Design review of the part built by this model. Coordinates are the model's own, in mm. A direction names the side the tool comes from. Coordinates: 2 decimals unless noted, no trailing zeros. Order: outer loops, then holes, each group sorted by start corner. A loop starts at its lowest first (then second) coordinate and runs counter-clockwise, first axis right, second up. Notation, with made-up numbers: M 85.25,24 L 135.25,24 A6 ccw 135.25,33 Z; hole C 84,9.5 d3. An arc over 180 degrees is marked long. Answer in a Markdown table with one row per item.
from build123d import *

# Parameters (mm, degrees)
F0_W      = 30
F0_H      = 45
F1_DEPTH  = 20
F2_W      = 6
F2_H      = 6
F3_DEPTH  = 1
F5_DEPTH  = 1
F6_W      = 1
F6_H      = 30
F7_DEPTH  = 30
F8_W      = 23
F8_H      = 23
F9_DEPTH  = 3
F10_W     = 23
F10_H     = 23
F11_DEPTH = 3
F12_W     = 42
F12_H     = 30
F13_DEPTH = 2
F14_R     = 8
F15_DEPTH = 8
F17_DEPTH = 15
F18_W     = 42
F18_H     = 22.5
F19_DEPTH = 14
F21_R     = 8
F22_DEPTH = 8
F23_DEPTH = 42
F24_DEPTH = 1
F25_R     = 8
F26_DEPTH = 8
F27_R     = 8
F28_DEPTH = 8
F29_W     = 6
F29_H     = 6
F30_DEPTH = 1
F31_W     = 42
F31_H     = 5
F32_DEPTH = 3


with BuildPart() as f1:
    # F0 (on Right) → F1 (new body, symmetric)
    with BuildSketch(Plane.YZ):
        Rectangle(F0_W, F0_H)
    extrude(amount=F1_DEPTH, both=True)

    # F2 (on face) → F3 (join, symmetric)
    with BuildSketch(Plane(origin=(-20, 0, 0), x_dir=(0, -1, 0), z_dir=(-1, 0, 0))):
        Polygon((-15, -7.5), (-15, -22.5), (15, -22.5), (15, -7.5), (4.0889219381, -7.5), (4.0889219381, 2.5), (-4.0889219381, 2.5), (-4.0889219381, -7.5), align=None)
        with Locations((-7.5, 10.5)):
            Rectangle(F2_W, F2_H)
        with Locations((7.5, 10.5)):
            Rectangle(F2_W, F2_H)
    extrude(amount=F3_DEPTH, both=True)

    # F4 (on face) → F5 (join, symmetric)
    with BuildSketch(Plane.YZ.offset(20)):
        Polygon((-4.0889219381, -7.5), (-15, -7.5), (-15, -22.5), (15, -22.5), (15, -7.5), (4.0889219381, -7.5), (4.0889219381, 2.5), (-4.0889219381, 2.5), align=None)
    extrude(amount=F5_DEPTH, both=True)

    # F6 (on face) → F7 (join)
    with BuildSketch(Plane(origin=(0, 15, 0), x_dir=(-1, 0, 0), z_dir=(0, 1, 0))):
        with Locations((20.5, 7.5)):
            Rectangle(F6_W, F6_H)
        Polygon((-21, -22.5), (21, -22.5), (21, -7.5), (20, -7.5), (20, 22.5), (-20, 22.5), (-20, -7.5), (-21, -7.5), align=None)
        with Locations((-20.5, 7.5)):
            Rectangle(F6_W, F6_H)
    extrude(amount=F7_DEPTH)

    # F8 (on face) → F9 (cut)
    with BuildSketch(Plane(origin=(-21, 0, 0), x_dir=(0, -1, 0), z_dir=(-1, 0, 0))):
        with Locations((-30, 7.5)):
            Rectangle(F8_W, F8_H)
    extrude(amount=-F9_DEPTH, mode=Mode.SUBTRACT)

    # F10 (on face) → F11 (cut)
    with BuildSketch(Plane.YZ.offset(21)):
        with Locations((30, 7.5)):
            Rectangle(F10_W, F10_H)
    extrude(amount=-F11_DEPTH, mode=Mode.SUBTRACT)

    # F12 (on face) → F13 (join)
    with BuildSketch(Plane.XY.offset(22.5)):
        with Locations((0, 30)):
            Rectangle(F12_W, F12_H)
    extrude(amount=F13_DEPTH)

    # F14 (on face) → F15 (cut)
    with BuildSketch(Plane(origin=(-21, 0, 0), x_dir=(0, -1, 0), z_dir=(-1, 0, 0))):
        with Locations((-27, -22.5)):
            Circle(F14_R)
    extrude(amount=-F15_DEPTH, mode=Mode.SUBTRACT)

    # F16 (on face) → F17 (join)
    with BuildSketch(Plane.XZ.offset(15)):
        Polygon((-21, 24.5194389681), (-21, -22.5), (21, -22.5), (21, 24.5022866875), align=None)
    extrude(amount=F17_DEPTH)

    # F18 (on face) → F19 (join)
    with BuildSketch(Plane.XZ.offset(30)):
        with Locations((0, -11.25)):
            Rectangle(F18_W, F18_H)
    extrude(amount=F19_DEPTH)

    # F21 (on face) → F22 (cut)
    with BuildSketch(Plane.YZ.offset(21)):
        with Locations((27, -22.5)):
            Circle(F21_R)
    extrude(amount=-F22_DEPTH, mode=Mode.SUBTRACT)

    # F20 (on face) → F23 (join)
    with BuildSketch(Plane(origin=(-21, 0, 0), x_dir=(0, -1, 0), z_dir=(-1, 0, 0))):
        Polygon((44, 0), (30, 24.5194389681), (30, 0), align=None)
    extrude(amount=-F23_DEPTH)

    # F2 (on face) → F24 (join)
    with BuildSketch(Plane(origin=(-20, 0, 0), x_dir=(0, -1, 0), z_dir=(-1, 0, 0))):
        Polygon((-15, -7.5), (-15, -22.5), (15, -22.5), (15, -7.5), (4.0889219381, -7.5), (4.0889219381, 2.5), (-4.0889219381, 2.5), (-4.0889219381, -7.5), align=None)
        with Locations((-7.5, 10.5)):
            Rectangle(F2_W, F2_H)
        with Locations((7.5, 10.5)):
            Rectangle(F2_W, F2_H)
    extrude(amount=F24_DEPTH)

    # F25 (on face) → F26 (cut)
    with BuildSketch(Plane(origin=(-21, 0, 0), x_dir=(0, -1, 0), z_dir=(-1, 0, 0))):
        with Locations((26, -22.5)):
            Circle(F25_R)
    extrude(amount=-F26_DEPTH, mode=Mode.SUBTRACT)

    # F27 (on face) → F28 (cut)
    with BuildSketch(Plane.YZ.offset(21)):
        with Locations((-28, -22.5)):
            Circle(F27_R)
    extrude(amount=-F28_DEPTH, mode=Mode.SUBTRACT)

    # F29 (on face) → F30 (join, symmetric)
    with BuildSketch(Plane.YZ.offset(20)):
        with Locations((-7.5, 10.5)):
            Rectangle(F29_W, F29_H)
        with Locations((7.5, 10.5)):
            Rectangle(F29_W, F29_H)
    extrude(amount=F30_DEPTH, both=True)

    # F31 (on face) → F32 (join)
    with BuildSketch(Plane.XZ.offset(44)):
        with Locations((0, -20)):
            Rectangle(F31_W, F31_H)
    extrude(amount=F32_DEPTH)


solid = f1.part
(1) Add section B-B, the plane z = -2.5. Give the boundary of the cut face in (x, y), and give its area (3 significant figures).
Return value:
| item | result |
|---|---|
| outline | M -21,-44 L 21,-44 L 21,-15 L 20,-15 L 20,-4.09 L 21,-4.09 L 21,4.09 L 20,4.09 L 20,15 L 21,15 L 21,18.5 L 18,18.5 L 18,41.5 L 21,41.5 L 21,45 L -21,45 L -21,41.5 L -18,41.5 L -18,18.5 L -21,18.5 L -21,15 L -20,15 L -20,4.09 L -21,4.09 L -21,-4.09 L -20,-4.09 L -20,-15 L -21,-15 Z |
| area | 3,560 mm2 |
(2) For line 1 along X through (y, z) = (35, 9); line 2 along Z through (x, y) = (-4, 41); line 3 along X through (y, z) = (-13.5, -6), list the stretches that pass through material, from the lowest coordinate up. Write a range as from..to.
Return value:
| item | result |
|---|---|
| line 1 | x = -18..18 |
| line 2 | z = -22.5..24.5 |
| line 3 | x = -20..20 |
(3) For faces 4 (the flat face through (20, 41.5, 7)), 5 (the flat face through (-20, 18.5, 7)), 6 (the flat face through (-13, -26, -19)), 7 (the flat face through (0, 15, 23)), 8 (the flat face through (13, -28, -19)), list the 3-axis set-ups (+Z, -Z, +X, -X, +Y, -Y) from which the entire face can be reached by the end or side of a thin tool; tool diameter is ignored.
Return value:
| item | result |
|---|---|
| face 4 | +X |
| face 5 | -X |
| face 6 | -Z, -X |
| face 7 | +Z |
| face 8 | -Z, +X |
(4) Add section D-D, the plane y = -1. Give the boundary of the cut face in (x, z), and give its area (3 significant figures).
Return value:
| item | result |
|---|---|
| outline | M -21,-22.5 L 21,-22.5 L 21,2.5 L 20,2.5 L 20,22.5 L -20,22.5 L -20,2.5 L -21,2.5 Z |
| area | 1,850 mm2 |
(5) Add section A-A, the plane y = 27. Give the boundary of the cut face in (x, z).
Return value:
| item | result |
|---|---|
| outline | M -21,-14.5 L -13,-14.5 L -13,-22.5 L 13,-22.5 L 13,-14.5 L 21,-14.5 L 21,-4 L 18,-4 L 18,19 L 21,19 L 21,24.5 L -21,24.5 L -21,19 L -18,19 L -18,-4 L -21,-4 Z |
(6) Draft analysis for pull direction Z (two halves, no side actions). For faces 1 (the cylindrical face through (-17.056, -26.176, -14.502)), 2 (the flat face through (-20, 30, 19)), 3 (the flat face through (0, -47, -20)), state which applies: pulls with the +Z half, pulls with the -Z half, needs draft (parallel to the pull), parting line crosses it, or undercut.
Return value:
| item | result |
|---|---|
| face 1 | pulls with the -Z half |
| face 2 | undercut |
| face 3 | needs draft |
(7) Insertion check: pin 1 Ø2 at (y, z) = (20.5, 6) entering from +X; pin 2 Ø0.8 at (x, z) = (-20.5, 9.5) entering from -Y; pin 3 Ø3 at (x, y) = (12.5, -22) entering from +Z. Each pin has a flat end and moves straight along its axis. Give the tip position at first contact, or say it passes through.
Return value:
| item | result |
|---|---|
| pin 1 | stops at x = 18 |
| pin 2 | stops at y = -38.8 |
| pin 3 | stops at z = 24.51 |
